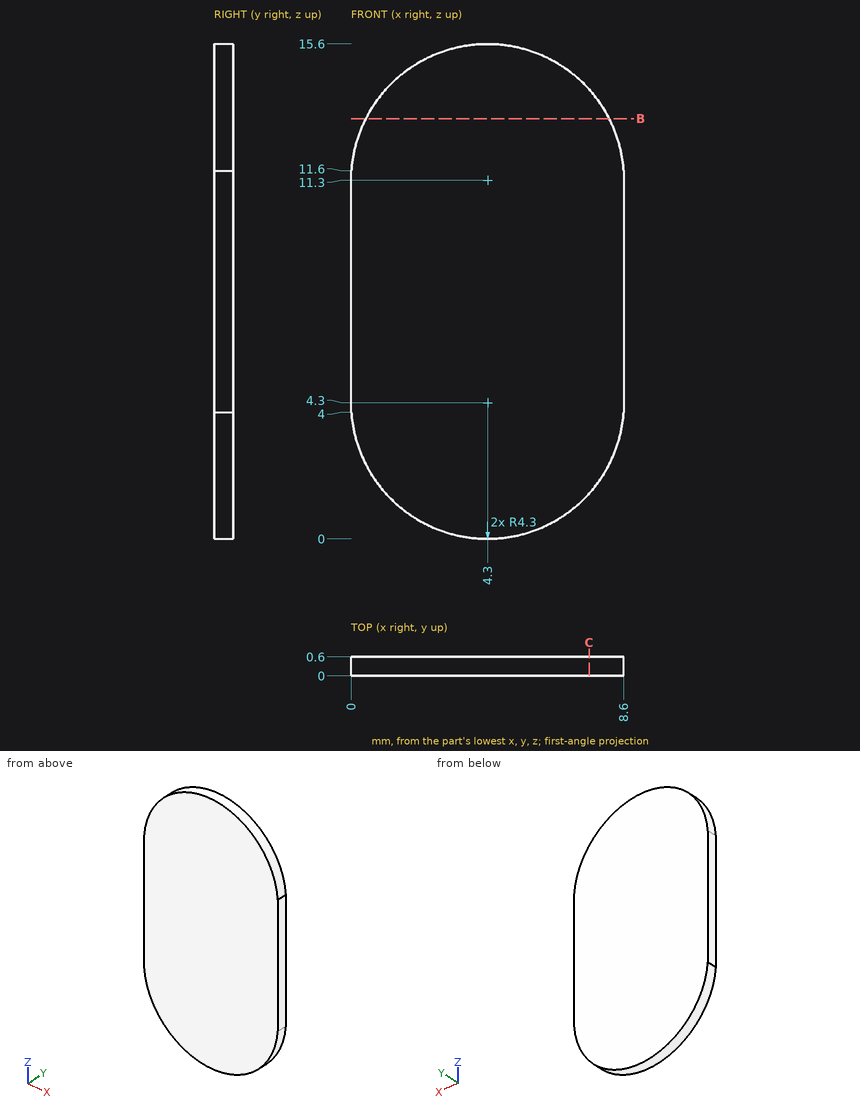
The figure shows three views and two pictorial views of one solid part (mm, origin at its lowest corner). Answer the questions. Coordinates: 2 decimals unless noted, no trailing zeros. Loops run counter-clockwise (first coordinate to the right, second up) from the corner with the lowest first, then second, coordinate; pieces in that order, holes last.
(1) Consider line 1 along Z through (x, y) = (1, 0.2); line 2 along X through (y, z) = (0.5, 15); line 3 along Z through (x, y) = (2.75, 0.05). Determine where each line is inside the solid, lowest interval first.
Solution:
line 1: z = 1.54 to 14.06
line 2: x = 2.11 to 6.49
line 3: z = 0.29 to 15.31
(2) The part is cut by section B-B (z = 13.25). Determine the outline of the cut face in (x, y), and give its area (3 significant figures).
Solution:
outline: (0.47, 0) - (8.13, 0) - (8.13, 0.6) - (0.47, 0.6) - close
area: 4.60 mm2
(3) The part is cut by section C-C (x = 7.5). Determine the outline of the cut face in (y, z).
Solution:
outline: (0, 1.43) - (0.6, 1.43) - (0.6, 14.17) - (0, 14.17) - close
(4) A flat-ended cylindrical pin translates along its axis: pin 1 Ø2 at (x, z) = (5.5, 10.5) entering from -Y. Find the tip coordinate at first contact, or state that the pin passes through.
Solution:
pin 1: stops at y = 0
